Here's how the part is built. I have some questions about the finished solid (model axes, mm). A direction names the side the tool comes from. Round coordinates to 2 decimals unless told otherwise and drop trailing zeros. Order: outer loops, then holes, each group sorted by start corner. A loop starts at its lowest first (then second) coordinate and runs counter-clockwise, first axis right, second up. Notation, with made-up numbers: M 71,5.5 L 113,5.5 A7 ccw 113,10.5 Z; hole C -26.75,-35 d11. An arc over 180 degrees is marked long. Write each question's results on one line, items separated by ' | '. Start each with the question number.
Autodesk Inventor part; units mm, degrees
ref_plane "YZ Plane" through (0, 0, 0) normal (1, 0, 0) x (0, 1, 0)
ref_plane "XZ Plane" through (0, 0, 0) normal (0, 1, 0) x (-1, 0, 0)
ref_plane "XY Plane" through (0, 0, 0) normal (0, 0, 1) x (1, 0, 0)
sketch "Sketch1" plane through (0, 0, 0) normal (0, 1, 0) x (-1, 0, 0)
  line L0 (-20.9775, 0) -> (0, 25)
  line L1 (0, 25) -> (20.9775, 0)
  line L2 (20.9775, 0) -> (-20.9775, 0)
  line L3 (0, 25) -> (0, 0) construction
  line L4 (0, 31.2229) -> (-29.5555, -4)
  line L5 (-29.5555, -4) -> (29.5555, -4)
  line L6 (29.5555, -4) -> (0, 31.2229)
  line L7 (27.206, -1.2) -> (-27.206, -1.2)
  dimension "d0" = 40
  dimension "d1" = 25
  dimension "d2" = 4
  dimension "d6" = 1.2
extrude "Extrusion1" add sketch "Sketch1" along normal blind 10 contours L6 L7 L4
fillet "Fillet1" radius 1 8 edges at (10.4887, 10, 12.5) (-10.4887, 10, 12.5) (-13.603, 0, 15.0114) (-10.4887, 0, 12.5) (-13.603, 10, 15.0114) (10.4887, 0, 12.5) (13.603, 0, 15.0114) (13.603, 10, 15.0114)
properties part number "test-triangle-overhang"
(1) Please list where these lines run through material, in increasing order: line 1 (Z direction, x = 16, y = 4.5); line 2 (Z direction, x = -19.5, y = 1.75); line 3 (X direction, y = 6.25, z = 0.5).
(2) I'm going to push flat-ended pins straight in: pin 1 Ø2 at (x, z) = (-8, 24) entering from +Y; pin 2 Ø3 at (x, y) = (6, 6.5) entering from +Z; pin 3 Ø3 at (y, z) = (2, 14) entering from +X; pin 4 Ø12 at (x, z) = (7, 8.5) entering from -Y. Where does each tip first touch, or does it pass through?
(3) On a 3-axis mill with a long thin cutter (end or side, diameter ignored), from which of +Z, -Z, +X, -X, +Y, -Y can I reach the whole of each face in a straight line? I mean faces 1 (the cylindrical face through (-10.76, 9.71, 12.64)), 2 (the flat face through (-10.342, 4.944, 12.675)), 3 (the cylindrical face through (10.44, 0.3, 13)). Say none if no direction works.
(4) If we mould it in two halves opening along Z, with no side actions, what happens to faces 4 (the cylindrical face through (10.45, 9.71, 13.01)), 5 (the cylindrical face through (13.563, 9.715, 14.591)), 6 (the flat face through (0, 5, -1.2))? For each: pulls with the +Z half, pulls with the -Z half, needs draft (parallel to the pull), parting line crosses it, or undercut.
(5) I want a section at A-A on y = 4.25. Write out the boundary of the cut face in (x, z), and give its area (3 significant figures).
Solutions:
1) line 1: -1.2 to 0, 5.93 to 12.15 | line 2: -1.2 to 0, 1.76 to 7.98 | line 3: -25.78 to -20.56, 20.56 to 25.78
2) pin 1: through | pin 2: z = 25.86 | pin 3: x = 15.71 | pin 4: y = 0.03
3) face 1: +Y | face 2: +Y, -Y | face 3: -Y
4) face 4: undercut | face 5: pulls with the +Z half | face 6: pulls with the -Z half
5) outline: M -27.21,-1.2 L 27.21,-1.2 L 0,31.22 Z; hole M -20.98,0 L 20.98,0 L 0,25 Z | area: 358 mm^2
